```python
from build123d import *

# Parameters (mm, degrees)
SKETCH1_R           = 7
BOSS_EXTRUDE1_DEPTH = 7
CUT_EXTRUDE1_START  = -7
CUT_EXTRUDE1_DEPTH  = 7
CIRPATTERN1_COUNT   = 20
SKETCH3_R           = 2.5
CUT_EXTRUDE2_DEPTH  = 7


with BuildPart() as part:
    # Sketch1 → Boss-Extrude1 (new body)
    with BuildSketch(Plane.XY):
        Circle(SKETCH1_R)
    extrude(amount=BOSS_EXTRUDE1_DEPTH)

    # Sketch2 → Cut-Extrude1 (cut)
    with BuildSketch(Plane.XY.offset(7).offset(CUT_EXTRUDE1_START)):
        with BuildLine():
            ThreePointArc((0.972302791, 6.1312752), (1.096934983, 6.541731598), (1.382072919, 6.862206238))
            ThreePointArc((1.382072919, 6.862206238), (0.549882168, 6.978368692), (-0.290231769, 6.993980663))
            ThreePointArc((-0.290231769, 6.993980663), (-0.058806828, 6.632801852), (0, 6.207890809))
            ThreePointArc((0, 6.207890809), (0.07898528, 5.889690377), (0.256638442, 5.614137219))
            ThreePointArc((0.256638442, 5.614137219), (0.441476826, 5.60263315), (0.62583581, 5.585045169))
            ThreePointArc((0.62583581, 5.585045169), (0.844454593, 5.829372853), (0.972302791, 6.1312752))
        make_face()
    cut_extrude1 = extrude(amount=CUT_EXTRUDE1_DEPTH, mode=Mode.SUBTRACT)

    # CirPattern1: Cut-Extrude1 ×20 about axis
    cirpattern1_axis = Axis((0, 0, 0), (0, 0, 1))
    for i in range(1, CIRPATTERN1_COUNT):
        add(cut_extrude1.rotate(cirpattern1_axis, i * 360 / CIRPATTERN1_COUNT), mode=Mode.SUBTRACT)

    # Sketch3 → Cut-Extrude2 (cut)
    with BuildSketch(Plane.XY.offset(7)):
        Circle(SKETCH3_R)
    extrude(amount=-CUT_EXTRUDE2_DEPTH, mode=Mode.SUBTRACT)

    # Sketch4 → Revolve3 (revolve)
    with BuildSketch(Plane(origin=(0, 0, 0), x_dir=(0, 0, -1), z_dir=(1, 0, 0)), mode=Mode.PRIVATE) as revolve3_sk:
        Polygon((0, -7.532770955), (0.125193645, -8), (0.511563976, -7.896472382), (0.4, -7.480109956), (0.4, -2.498650108), (0, -2.498650108), align=None)
    revolve(revolve3_sk.sketch.rotate(Axis((0, 0, 0), (0, 0, -1)), 270), axis=Axis((0, 0, 0), (0, 0, -1)))

    # Sketch7 → Revolve4 (revolve)
    with BuildSketch(Plane(origin=(0, 0, 0), x_dir=(0, 0, -1), z_dir=(1, 0, 0)), mode=Mode.PRIVATE) as revolve4_sk:
        Polygon((-7, 3.370594433), (-7, 7.532770955), (-7.125193645, 8), (-15.235193645, 8), (-15.485193645, 7.75), (-15.485193645, 3.370594433), align=None)
    revolve(revolve4_sk.sketch.rotate(Axis((0, -0.003090187, 7), (0, 0, 1)), 90), axis=Axis((0, -0.003090187, 7), (0, 0, 1)))


solid = part.part
```
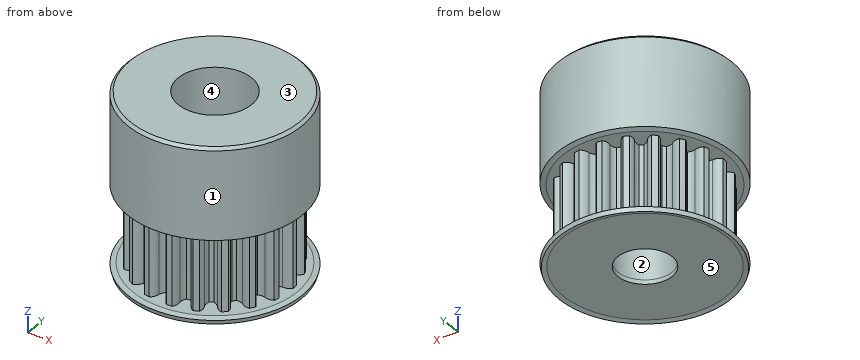
CAD build for the part. Positions are in the model's coordinates, mm. Face numbers are marked on the shaded views. A direction names the side the tool comes from. Round coordinates to 2 decimals unless told otherwise and drop trailing zeros. Order: outer loops, then holes, each group sorted by start corner. A loop starts at its lowest first (then second) coordinate and runs counter-clockwise, first axis right, second up.
Item 1: Pin check, flat tips, straight feed: pin 1 (3 mm diameter, centred on x = 3, z = 2.5, fed in from +Y); pin 2 (9 mm diameter, centred on x = 0, y = 0, fed in from +Z); pin 3 (2.5 mm diameter, centred on x = 0, y = -0.5, fed in from +Z); pin 4 (2 mm diameter, centred on x = -6, z = 10.5, fed in from +Y). Stop position of each tip, or through.
Item 2: Saw through at A-A on z = 11. Write the cut outline in (x, y), then the cut area to 3 significant figures.
Item 3: Tool access for the marked faces 4 and 5: list every direction of +Z, -Z, +X, -X, +Y, -Y with a clear straight run to the whole face (end or side of a thin tool).
Item 4: Probe line 1 along Y through (x, z) = (0, 10.75); line 2 along Y through (x, z) = (6, 4); line 3 along Z through (x, y) = (-3.75, -4.5). List the from-to ranges inside material, lowest first.
Item 5: Mould opens along X. For the marked faces 1, 2 and 3 say: pulls with the +X half, pulls with the -X half, needs draft (parallel to the pull), parting line crosses it, or undercut.
Reported:
1. pin 1: stops at y = 6.84
1. pin 2: stops at z = 15.49
1. pin 3: passes through
1. pin 4: stops at y = 6.25
2. outline: circle Ø16.01 at (0, 0); hole circle Ø6.75 at (0, 0)
2. area: 165 mm2
3. face 4: +Z
3. face 5: -Z
4. line 1: y = -8.01 to -3.38, 3.37 to 8
4. line 2: y = -3.61 to -3.22, -1.95 to -0.93, -0.04 to 0.97, 1.95 to 2.96
4. line 3: z = -0.4 to 0, 7 to 15.49
5. face 1: parting line crosses it
5. face 2: undercut
5. face 3: needs draft
